Model file for the job. Use its own axes, mm. A direction names the side the tool comes from. Give positions to 0.01 mm unless a question says otherwise; leave off trailing zeros. Order: outer loops, then holes, each group sorted by start corner. A loop starts at its lowest first (then second) coordinate and runs counter-clockwise, first axis right, second up. Notation, with made-up numbers: M -2.75,-12 L 28.25,-12 A22 ccw 28.25,-3 Z; hole C 13.25,11 d10. An arc over 180 degrees is marked long. Return JSON: item names as keys, results as strings. Group by question number.
1. Pin check, flat tips, straight feed: pin 1 (1.3 mm diameter, centred on x = 25.5, z = 14.5, fed in from +Y); pin 2 (1.5 mm diameter, centred on x = -3, z = -9.5, fed in from -Y); pin 3 (0.8 mm diameter, centred on x = 0, z = 11, fed in from -Y). Stop position of each tip, or through.
2. Slice it at A-A on y = 20. Give the number of separate pieces and of enclosed holes in the cut face, then the cut area to 3 significant figures.
3. Two-plate mould, pull along X, no slides. Class faces 1 (the face through (-24, 22.8, -8)), 2 (the face through (26.578, 18.876, -7.762)): released by +X, released by -X, zero draft, split by the parting line, or undercut.
4. Slice it at B-B on x = 0. List the corners of the cut face in (y, z).
5. 3-axis set-ups, long thin cutter, end or side, ignore diameter. For faces 3 (the face through (-21.422, 18.876, 8.238)), 4 (the face through (25.6, 4, 15.8)), 5 (the face through (18.501, 4, 15)): which of +Z, -Z, +X, -X, +Y, -Y reach the whole face in a straight line?
6. Wall check: probe 1 along X at (y, z) = (13.5, -11); probe 2 along X at (y, z) = (18.9, -8.1); probe 3 along X at (y, z) = (4.5, -9.5). Give the ranges that are in metal, low to high. Write a range as [from, to].
from build123d import *

# Parameters (mm, degrees)
SKETCH1_W               = 63.6
SKETCH1_H               = 31.6
BOSS_EXTRUDE1_DEPTH     = 19.2
SKETCH2_W               = 58.8
SKETCH2_H               = 26.8
CUT_EXTRUDE1_DEPTH      = 17.2
SKETCH3_R               = 4.8
BOSS_EXTRUDE2_DEPTH     = 3.6
LPATTERN1_COUNT         = 4
LPATTERN1_PITCH         = 16
LPATTERN1_COUNT_DIR2    = 2
LPATTERN1_PITCH_DIR2    = 16
SKETCH4_R               = 2.6
CUT_EXTRUDE2_DEPTH      = 3.4
LPATTERN2_COUNT         = 4
LPATTERN2_PITCH         = 16
LPATTERN2_COUNT_DIR2    = 2
LPATTERN2_PITCH_DIR2    = 16
SKETCH5_R               = 6.51
SKETCH5_R_2             = 4.8
BOSS_EXTRUDE3_DEPTH     = 17.2
LPATTERN3_COUNT         = 2
LPATTERN3_PITCH         = 16
LPATTERN4_COUNT         = 2
LPATTERN4_PITCH         = 16
BOSS_EXTRUDE4_DEPTH     = 12.6
BOSS_EXTRUDE5_REACH     = 44.199
SKETCH7_R               = 0.6
LPATTERN5_COUNT         = 4
LPATTERN5_PITCH         = 16
SKETCH8_R               = 0.6
BOSS_EXTRUDE6_DEPTH     = 17.2
MIRROR2_COPY_1_REACH    = 44.199
MIRROR2_COPY_1_SKETCH_R = 0.6
MIRROR2_COPY_2_REACH    = 44.199
MIRROR2_COPY_2_SKETCH_R = 0.6
MIRROR2_COPY_3_REACH    = 44.199
MIRROR2_COPY_3_SKETCH_R = 0.6
SKETCH9_W               = 0.314102564
SKETCH9_H               = 3.5
CUT_EXTRUDE3_DEPTH      = 2
SKETCH10_R              = 0.6
BOSS_EXTRUDE7_DEPTH     = 17.2


with BuildPart() as part:
    # Sketch1 → Boss-Extrude1 (new body)
    with BuildSketch(Plane(origin=(0, 0, 0), x_dir=(1, 0, 0), z_dir=(0, 1, 0))):
        Rectangle(SKETCH1_W, SKETCH1_H)
    extrude(amount=BOSS_EXTRUDE1_DEPTH)

    # Sketch2 → Cut-Extrude1 (cut)
    with BuildSketch(Plane.XZ):
        Rectangle(SKETCH2_W, SKETCH2_H)
    extrude(amount=-CUT_EXTRUDE1_DEPTH, mode=Mode.SUBTRACT)

    # Sketch3 → Boss-Extrude2 (add)
    with BuildSketch(Plane(origin=(0, 19.2, 0), x_dir=(1, 0, 0), z_dir=(0, 1, 0))):
        with Locations(Location((24, 7.9, 0), (0, 0, 90))):
            Circle(SKETCH3_R)
    boss_extrude2 = extrude(amount=BOSS_EXTRUDE2_DEPTH)

    # LPattern1: Boss-Extrude2 4 × 2
    with Locations(*[(-i * LPATTERN1_PITCH, 0, j * LPATTERN1_PITCH_DIR2) for i in range(LPATTERN1_COUNT) for j in range(LPATTERN1_COUNT_DIR2) if (i, j) != (0, 0)]):
        add(boss_extrude2)

    # Sketch4 → Cut-Extrude2 (cut)
    with BuildSketch(Plane(origin=(0, 17.2, 0), x_dir=(-1, 0, 0), z_dir=(0, -1, 0))):
        with Locations(Location((-24, -7.9, 0), (0, 0, 90))):
            Circle(SKETCH4_R)
    cut_extrude2 = extrude(amount=-CUT_EXTRUDE2_DEPTH, mode=Mode.SUBTRACT)

    # LPattern2: Cut-Extrude2 4 × 2
    with Locations(*[(-i * LPATTERN2_PITCH, 0, -j * LPATTERN2_PITCH_DIR2) for i in range(LPATTERN2_COUNT) for j in range(LPATTERN2_COUNT_DIR2) if (i, j) != (0, 0)]):
        add(cut_extrude2, mode=Mode.SUBTRACT)

    # Sketch5 → Boss-Extrude3 (add)
    with BuildSketch(Plane.XZ.offset(-17.2)):
        with Locations(Location((0, 0, 0), (0, 0, 270))):
            Circle(SKETCH5_R)
        with Locations(Location((0, 0, 0), (0, 0, 270))):
            Circle(SKETCH5_R_2, mode=Mode.SUBTRACT)
    boss_extrude3 = extrude(amount=BOSS_EXTRUDE3_DEPTH)

    # LPattern3: Boss-Extrude3 ×2
    with Locations(*[(i * LPATTERN3_PITCH, 0, 0) for i in range(1, LPATTERN3_COUNT)]):
        add(boss_extrude3)

    # LPattern4: Boss-Extrude3 ×2
    with Locations(*[(-i * LPATTERN4_PITCH, 0, 0) for i in range(1, LPATTERN4_COUNT)]):
        add(boss_extrude3)

    # Sketch6 → Boss-Extrude4 (add)
    with BuildSketch(Plane.XZ.offset(-17.2)):
        with BuildLine():
            Line((0.8, 13.4), (0, 13.4))
            Line((0, 13.4), (0, 6.51))
            ThreePointArc((0, 6.51), (0.400760105, 6.497652756), (0.8, 6.460657861))
            Line((0.8, 6.460657861), (0.8, 13.4))
        make_face()
        with BuildLine():
            Line((0, 6.51), (0, 13.4))
            Line((0, 13.4), (-0.8, 13.4))
            Line((-0.8, 13.4), (-0.8, 6.460657861))
            ThreePointArc((-0.8, 6.460657861), (-0.400760105, 6.497652756), (0, 6.51))
        make_face()
        with BuildLine():
            Line((0, -13.4), (0, -6.51))
            ThreePointArc((0, -6.51), (-0.400760105, -6.497652756), (-0.8, -6.460657861))
            Line((-0.8, -6.460657861), (-0.8, -13.4))
            Line((-0.8, -13.4), (0, -13.4))
        make_face()
        with BuildLine():
            ThreePointArc((0.8, -6.460657861), (0.400760105, -6.497652756), (0, -6.51))
            Line((0, -6.51), (0, -13.4))
            Line((0, -13.4), (0.8, -13.4))
            Line((0.8, -13.4), (0.8, -6.460657861))
        make_face()
    extrude(amount=BOSS_EXTRUDE4_DEPTH)

    # Sketch7 → Boss-Extrude5 (add, up to next)
    with BuildSketch(Plane.XZ, mode=Mode.PRIVATE) as boss_extrude5_sk1:
        with Locations((24, 13.4)):
            Circle(SKETCH7_R)
    boss_extrude5_tool1 = extrude(boss_extrude5_sk1.sketch, amount=-BOSS_EXTRUDE5_REACH, mode=Mode.PRIVATE) - part.part
    boss_extrude5 = boss_extrude5_tool1.solids().sort_by_distance((24, 0, 13.4))[0]
    add(boss_extrude5)

    # LPattern5: Boss-Extrude5 ×4
    with Locations(*[(-i * LPATTERN5_PITCH, 0, 0) for i in range(1, LPATTERN5_COUNT)]):
        add(boss_extrude5)

    # Sketch8 → Boss-Extrude6 (add)
    with BuildSketch(Plane(origin=(0, 0, 0), x_dir=(-1, 0, 0), z_dir=(0, -1, 0))):
        with Locations((-29.4, -7.9)):
            Circle(SKETCH8_R)
    boss_extrude6 = extrude(amount=-BOSS_EXTRUDE6_DEPTH)

    # Mirror2: Boss-Extrude5 across plane
    add(boss_extrude5.mirror(Plane.XY))

    # Mirror2 copy 1 sketch → Mirror2 copy 1 (add, up to next)
    with BuildSketch(Plane(origin=(-16, 0, 0), x_dir=(1, 0, 0), z_dir=(0, -1, 0)), mode=Mode.PRIVATE) as mirror2_copy_1_sk1:
        with Locations((24, -13.4)):
            Circle(MIRROR2_COPY_1_SKETCH_R)
    mirror2_copy_1_tool1 = extrude(mirror2_copy_1_sk1.sketch, amount=-MIRROR2_COPY_1_REACH, mode=Mode.PRIVATE) - part.part
    add(mirror2_copy_1_tool1.solids().sort_by_distance((8, 0, -13.4))[0])

    # Mirror2 copy 2 sketch → Mirror2 copy 2 (add, up to next)
    with BuildSketch(Plane(origin=(-32, 0, 0), x_dir=(1, 0, 0), z_dir=(0, -1, 0)), mode=Mode.PRIVATE) as mirror2_copy_2_sk1:
        with Locations((24, -13.4)):
            Circle(MIRROR2_COPY_2_SKETCH_R)
    mirror2_copy_2_tool1 = extrude(mirror2_copy_2_sk1.sketch, amount=-MIRROR2_COPY_2_REACH, mode=Mode.PRIVATE) - part.part
    add(mirror2_copy_2_tool1.solids().sort_by_distance((-8, 0, -13.4))[0])

    # Mirror2 copy 3 sketch → Mirror2 copy 3 (add, up to next)
    with BuildSketch(Plane(origin=(-48, 0, 0), x_dir=(1, 0, 0), z_dir=(0, -1, 0)), mode=Mode.PRIVATE) as mirror2_copy_3_sk1:
        with Locations((24, -13.4)):
            Circle(MIRROR2_COPY_3_SKETCH_R)
    mirror2_copy_3_tool1 = extrude(mirror2_copy_3_sk1.sketch, amount=-MIRROR2_COPY_3_REACH, mode=Mode.PRIVATE) - part.part
    add(mirror2_copy_3_tool1.solids().sort_by_distance((-24, 0, -13.4))[0])

    # Sketch9 → Cut-Extrude3 (cut)
    # profile 1 of 4: a face of its own
    with BuildSketch(Plane.XY.offset(15.8)):
        Polygon((15.808248921, 2), (15.808248921, 5.5), (15.87415437, 5.5), (18.186454049, 2.745292468), (18.186454049, 5.5), (18.500556613, 5.5), (18.500556613, 2), (18.42904219, 2), (16.122351485, 4.748397436), (16.122351485, 2), align=None)
    # profile 2 of 4: a face of its own
    with BuildSketch(Plane.XY.offset(15.8)):
        with Locations((19.555043793, 3.75)):
            Rectangle(SKETCH9_W, SKETCH9_H)
    # profile 3 of 4: a face of its own
    with BuildSketch(Plane.XY.offset(15.8)):
        Polygon((20.609530972, 2), (20.609530972, 5.5), (20.675436421, 5.5), (22.987736101, 2.745292468), (22.987736101, 5.5), (23.301838665, 5.5), (23.301838665, 2), (23.230324242, 2), (20.923633537, 4.748397436), (20.923633537, 2), align=None)
    # profile 4 of 4: a face of its own
    with BuildSketch(Plane.XY.offset(15.8)):
        Polygon((25.635171998, 5.5), (27.250556613, 2), (26.909110299, 2), (26.391682415, 3.121794872), (24.805043793, 3.121794872), (24.273593472, 2), (23.930043793, 2), (25.590300203, 5.5), align=None)
        Polygon((25.609230492, 4.817107372), (24.976117511, 3.480769231), (26.226217671, 3.480769231), align=None, mode=Mode.SUBTRACT)
    extrude(amount=-CUT_EXTRUDE3_DEPTH, mode=Mode.SUBTRACT)

    # Sketch10 → Boss-Extrude7 (add)
    with BuildSketch(Plane(origin=(0, 0, 0), x_dir=(-1, 0, 0), z_dir=(0, -1, 0))):
        with Locations((-29.4, 7.9)):
            Circle(SKETCH10_R)
    boss_extrude7 = extrude(amount=-BOSS_EXTRUDE7_DEPTH)

    # Mirror3: Boss-Extrude6, Boss-Extrude7 across plane
    add(boss_extrude6.mirror(Plane(origin=(0, 0, 0), x_dir=(0, 0, 1), z_dir=(1, 0, 0))))
    add(boss_extrude7.mirror(Plane(origin=(0, 0, 0), x_dir=(0, 0, 1), z_dir=(1, 0, 0))))


solid = part.part
Result:
{
 "1": {"pin 1": "stops at y = 19.2", "pin 2": "stops at y = 17.2", "pin 3": "stops at y = 4.6"},
 "2": {"separate pieces": "8", "enclosed holes": "8", "area": "409 mm2"},
 "3": {"face 1": "zero draft", "face 2": "undercut"},
 "4": {"outline": "M 0,-15.8 L 19.2,-15.8 L 19.2,15.8 L 0,15.8 L 0,13.4 L 4.6,13.4 L 4.6,6.51 L 0,6.51 L 0,4.8 L 17.2,4.8 L 17.2,-4.8 L 0,-4.8 L 0,-6.51 L 4.6,-6.51 L 4.6,-13.4 L 0,-13.4 Z"},
 "5": {"face 3": "-Y", "face 4": "+Z, +X, -X, +Y, -Y", "face 5": "+Z"},
 "6": {"probe 1": "x = [-31.8, -29.4], [-0.8, 0.8], [29.4, 31.8]", "probe 2": "x = [-31.8, -26.6], [-21.4, -10.6], [-5.4, 5.4], [10.6, 21.4], [26.6, 31.8]", "probe 3": "x = [-31.8, -29.4], [29.4, 31.8]"}
}
